Model file for the job. Use its own axes, mm. Face numbers are marked on the shaded views. A direction names the side the tool comes from. Give positions to 0.01 mm unless a question says otherwise; leave off trailing zeros. Loops run counter-clockwise (first coordinate to the right, second up) from the corner with the lowest first, then second, coordinate; pieces in that order, holes last. Notation, with made-up numbers: M -13.75,21.25 L 17.25,21.25 A24 ccw 17.25,60.25 Z; hole C 39.25,77.25 d2. An arc over 180 degrees is marked long. Answer in a Markdown table with one row per item.
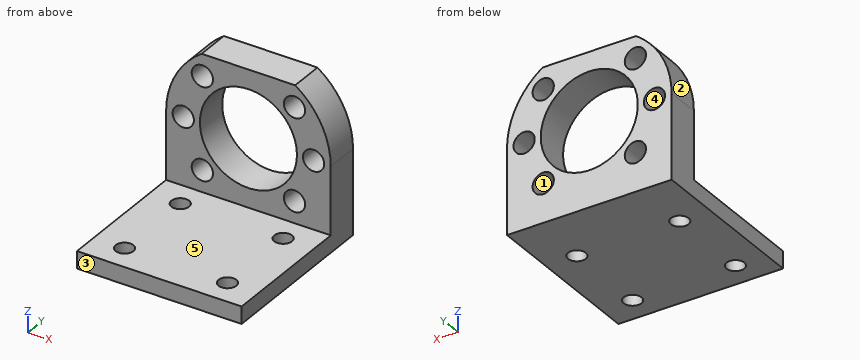
```python
from build123d import *

# Parameters (mm, degrees)
F0_R     = 3.1
F0_R_2   = 14.15
F1_DEPTH = 10
F2_W     = 48
F2_H     = 5
F3_DEPTH = 40
F4_R     = 2.6
F5_DEPTH = 5


with BuildPart() as f1:
    # F0 (on Front) → F1 (new body)
    with BuildSketch(Plane.XZ):
        with BuildLine():
            Line((13.63589, 19.75), (-13.63589, 19.75))
            ThreePointArc((-13.63589, 19.75), (-21.251604, 11.152099), (-24, 0))
            Line((-24, 0), (-24, -24.75))
            Line((-24, -24.75), (24, -24.75))
            Line((24, -24.75), (24, 0))
            ThreePointArc((24, 0), (21.251604, 11.152099), (13.63589, 19.75))
        make_face()
        with Locations((-13.435029, -13.435029)):
            Circle(F0_R, mode=Mode.SUBTRACT)
        with Locations((13.435029, -13.435029)):
            Circle(F0_R, mode=Mode.SUBTRACT)
        with Locations((-19, 0)):
            Circle(F0_R, mode=Mode.SUBTRACT)
        with Locations((-13.435029, 13.435029)):
            Circle(F0_R, mode=Mode.SUBTRACT)
        Circle(F0_R_2, mode=Mode.SUBTRACT)
        with Locations((19, 0)):
            Circle(F0_R, mode=Mode.SUBTRACT)
        with Locations((13.435029, 13.435029)):
            Circle(F0_R, mode=Mode.SUBTRACT)
    extrude(amount=F1_DEPTH)

    # F2 (on face) → F3 (join)
    with BuildSketch(Plane.XZ.offset(10)):
        with Locations((0, -22.25)):
            Rectangle(F2_W, F2_H)
    extrude(amount=F3_DEPTH)

    # F4 (on face) → F5 (cut, through all)
    with BuildSketch(Plane.XY.offset(-19.75)):
        with Locations((-15, -17.5)):
            Circle(F4_R)
        with Locations((-15, -42.5)):
            Circle(F4_R)
        with Locations((15, -42.5)):
            Circle(F4_R)
        with Locations((15, -17.5)):
            Circle(F4_R)
    extrude(amount=-F5_DEPTH, mode=Mode.SUBTRACT)


solid = f1.part
```
(1) Saw through at D-D, the plane x = 11. Give the cut face in (y, z), and give its area (3 significant figures).
Established:
| item | result |
|---|---|
| outline | M -50,-24.75 L 0,-24.75 L 0,-15.35 L -10,-15.35 L -10,-19.75 L -50,-19.75 Z; M -10,-11.52 L 0,-11.52 L 0,-8.9 L -10,-8.9 Z; M -10,8.9 L 0,8.9 L 0,11.52 L -10,11.52 Z; M -10,15.35 L 0,15.35 L 0,19.75 L -10,19.75 Z |
| area | 390 mm2 |
(2) Saw through at A-A, the plane y = -42.5. Give the cut face in (x, z), and give its area (3 significant figures).
Established:
| item | result |
|---|---|
| outline | M -24,-24.75 L -17.6,-24.75 L -17.6,-19.75 L -24,-19.75 Z; M -12.4,-24.75 L 12.4,-24.75 L 12.4,-19.75 L -12.4,-19.75 Z; M 17.6,-24.75 L 24,-24.75 L 24,-19.75 L 17.6,-19.75 Z |
| area | 188 mm2 |
(3) Saw through at C-C, the plane z = -9. Give the cut face in (x, y), and give its area (3 significant figures).
Established:
| item | result |
|---|---|
| outline | M -24,-10 L -10.92,-10 L -10.92,0 L -24,0 Z; M 10.92,-10 L 24,-10 L 24,0 L 10.92,0 Z |
| area | 262 mm2 |
(4) Flat gauge pins, fed straight in: P1, Ø4, axis at x = -15, y = -17.5, coming from the +Z side; P2, Ø2, axis at x = -13, y = -14.5, coming from the +Z side. Where does each tip first touch, or does it go through?
Established:
| item | result |
|---|---|
| P1 | passes through |
| P2 | stops at z = -19.75 |
(5) Wall check: L1, parallel to Y at x = -15, z = -21.4; L2, parallel to Y at x = 13, z = -21; L3, parallel to X at y = -42, z = -21. Give the ranges that are in metal, low to high.
Established:
| item | result |
|---|---|
| L1 | y = -50 to -45.1, -39.9 to -20.1, -14.9 to 0 |
| L2 | y = -50 to -44.16, -40.84 to -19.16, -15.84 to 0 |
| L3 | x = -24 to -17.55, -12.45 to 12.45, 17.55 to 24 |
(6) Mould opens along Z. For the marked faces 1, 2 and 3 say: pulls with the +Z half, pulls with the -Z half, needs draft (parallel to the pull), parting line crosses it, or undercut.
Established:
| item | result |
|---|---|
| face 1 | undercut |
| face 2 | pulls with the +Z half |
| face 3 | needs draft |
(7) Saw through at B-B, the plane x = 0. Give the cut face in (y, z), and give its area (3 significant figures).
Established:
| item | result |
|---|---|
| outline | M -50,-24.75 L 0,-24.75 L 0,-14.15 L -10,-14.15 L -10,-19.75 L -50,-19.75 Z; M -10,14.15 L 0,14.15 L 0,19.75 L -10,19.75 Z |
| area | 362 mm2 |
(8) Which spindle directions (+Z, -Z, +X, -X, +Y, -Y) get a long thin tool onto all of the face, cutting with end or side? Do the marked faces 4 and 5. Say none if no direction does.
Established:
| item | result |
|---|---|
| face 4 | +Y, -Y |
| face 5 | +Z, +X, -X, -Y |
